The figure shows three views and two pictorial views of one solid part (mm, origin at its lowest corner). Answer the questions. Round coordinates to 2 decimals unless told otherwise and drop trailing zeros. Loops run counter-clockwise (first coordinate to the right, second up) from the corner with the lowest first, then second, coordinate; pieces in that order, holes last. Notation, with made-up numbers: (81.25, 89.25) - (125.25, 89.25) arc R17 ccw to (125.25, 122.25) - close; hole circle Ø11 at (28, 17). An arc over 180 degrees is marked (long way). Use one line per item in the form item = value. Start each with the question number.
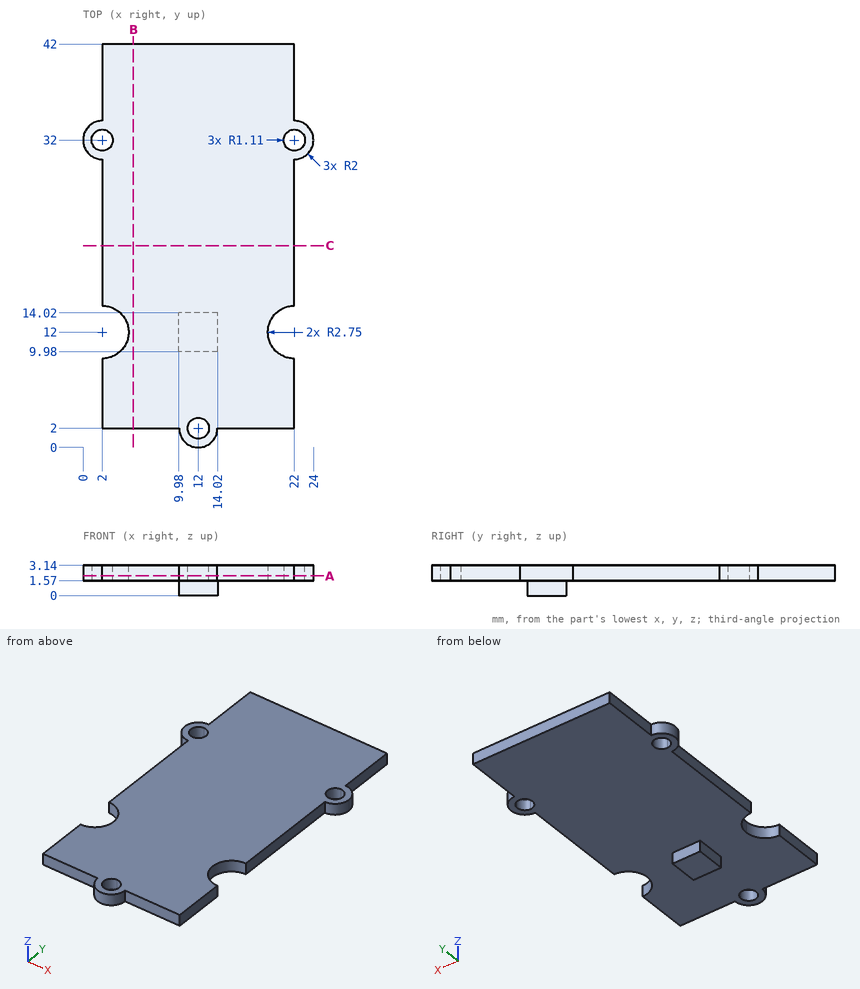
1) A cutting plane is placed at A-A on z = 2.05. Write down the section's boundary in (x, y).
2) Straight lines are drawn through the part: line 1 (Z direction, x = 8.5, y = 22.5); line 2 (X direction, y = 18, z = 2.8); line 3 (Y direction, x = 21.25, z = 2.05) (1 decimal). For each, find the intervals that lie inside material, in ascending order. Write a range as from..to.
3) A cutting plane is placed at B-B on x = 5.25. Write down the section's boundary in (y, z).
4) Flat-ended cylindrical pins translate along their axes: pin 1 (6 mm diameter, centred on x = 18, y = 37, fed in from -Z); pin 2 (1.7 mm diameter, centred on y = 20, z = 2.5, fed in from -X); pin 3 (0.5 mm diameter, centred on x = 12, z = 1, fed in from +Y). Find the tip coordinate at first contact, or state that the pin passes through.
5) A cutting plane is placed at C-C on y = 21. Write down the section's boundary in (x, z).
Checks:
q1.outline = (2, 2) - (10, 2) arc R2 ccw to (14, 2) - (22, 2) - (22, 9.25) arc R2.75 cw to (22, 14.75) - (22, 30) arc R2 ccw to (22, 34) - (22, 42) - (2, 42) - (2, 34) arc R2 ccw to (2, 30) - (2, 14.75) arc R2.75 cw to (2, 9.25) - close; hole circle Ø2.22 at (2, 32); hole circle Ø2.22 at (12, 2); hole circle Ø2.22 at (22, 32)
q2.line_1 = 1.57..3.14
q2.line_2 = 2..22
q2.line_3 = 2..9.4, 14.6..31.2, 32.8..42
q3.outline = (2, 1.57) - (42, 1.57) - (42, 3.14) - (2, 3.14) - close
q4.pin_1 = 1.57
q4.pin_2 = 2
q4.pin_3 = 14.02
q5.outline = (2, 1.57) - (22, 1.57) - (22, 3.14) - (2, 3.14) - close
